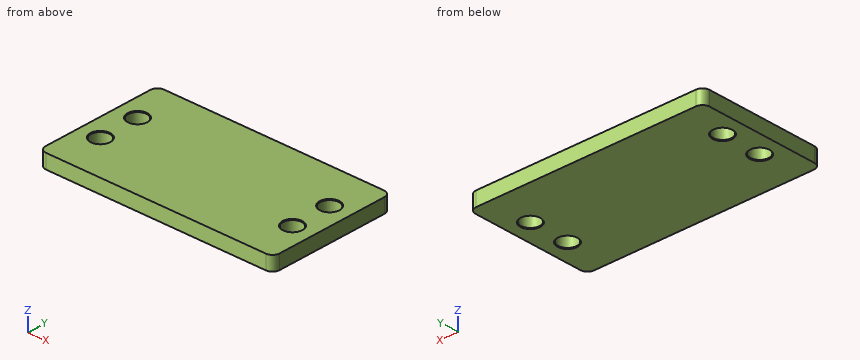
from build123d import *

# Parameters (mm, degrees)
SKETCH1_W                                 = 104.775
SKETCH1_H                                 = 57.15
BOSS_EXTRUDE1_DEPTH                       = 6.35
F_21_64_0_32813_DIAMETER_HOLE1_AT_2_COUNT = 2
F_21_64_0_32813_DIAMETER_HOLE1_AT_2_PITCH = 18
FILLET1_R                                 = 3.175


with BuildPart() as part:
    # Sketch1 → Boss-Extrude1 (new body)
    with BuildSketch(Plane.XY):
        Rectangle(SKETCH1_W, SKETCH1_H)
    extrude(amount=-BOSS_EXTRUDE1_DEPTH)

    # Sketch2 → 21/64 (0.32813) Diameter Hole1 (revolve, cut)
    with BuildSketch(Plane(origin=(43.000000106, 9, 0), x_dir=(0, -1, 0), z_dir=(1, 0, 0))):
        Polygon((0, 0), (0, 6.35), (4.445, 6.35), (4.167251, 6.072251), (4.167251, 0.277749), (4.445, 0), align=None)
    f_21_64_0_32813_diameter_hole1 = revolve(axis=Axis((43.000000106, 9, 6.35), (0, 0, -1)), mode=Mode.SUBTRACT)

    # 21/64 (0.32813) Diameter Hole1 at 2: 21/64 (0.32813) Diameter Hole1 ×2
    with Locations(*[(0, -i * F_21_64_0_32813_DIAMETER_HOLE1_AT_2_PITCH, 0) for i in range(1, F_21_64_0_32813_DIAMETER_HOLE1_AT_2_COUNT)]):
        add(f_21_64_0_32813_diameter_hole1, mode=Mode.SUBTRACT)

    # Mirror1: 21/64 (0.32813) Diameter Hole1 across plane
    add(f_21_64_0_32813_diameter_hole1.mirror(Plane(origin=(0, 0, 0), x_dir=(0, 0, 1), z_dir=(1, 0, 0))), mode=Mode.SUBTRACT)

    # Mirror1 copy 1 sketch → Mirror1 copy 1 (revolve, cut)
    with BuildSketch(Plane(origin=(-43.000000106, -9, 0), x_dir=(0, -1, 0), z_dir=(-1, 0, 0))):
        Polygon((0, 0), (0, -6.35), (4.445, -6.35), (4.167251, -6.072251), (4.167251, -0.277749), (4.445, 0), align=None)
    revolve(axis=Axis((-43.000000106, -9, 6.35), (0, 0, 1)), mode=Mode.SUBTRACT)

    # Fillet1
    fillet1_edges = [part.edges().sort_by_distance(p)[0] for p in [
        (-52.3875, 28.575, -3.175),
        (52.3875, 28.575, -3.175),
        (52.3875, -28.575, -3.175),
        (-52.3875, -28.575, -3.175),
    ]]
    fillet(fillet1_edges, radius=FILLET1_R)


solid = part.part
Part model, mm, in its own coordinate system. Coordinates: 2 decimals unless noted, no trailing zeros. Order: outer loops, then holes, each group sorted by start corner. A loop starts at its lowest first (then second) coordinate and runs counter-clockwise, first axis right, second up. Notation, with made-up numbers: M 55.25,64 L 62.25,64 A18 cw 62.25,85 Z; hole C 47.25,55 d4. An arc over 180 degrees is marked long. Use a Markdown table: item, result.
(1) Cut at B-B on x = 43. Write the cut outline in (y, z) (3 decimals), then the cut area to 3 significant figures.
A:
| item | result |
|---|---|
| outline | M -28.575,-6.35 L -13.445,-6.35 L -13.167,-6.072 L -13.167,-0.278 L -13.445,0 L -28.575,0 Z; M -4.833,-6.072 L -4.555,-6.35 L 4.555,-6.35 L 4.833,-6.072 L 4.833,-0.278 L 4.555,0 L -4.555,0 L -4.833,-0.278 Z; M 13.167,-6.072 L 13.445,-6.35 L 28.575,-6.35 L 28.575,0 L 13.445,0 L 13.167,-0.278 Z |
| area | 257 mm^2 |
(2) Cut at A-A on y = 9. State how many separate pieces and enclosed holes the cut face has, then the cut area to 3 significant figures.
A:
| item | result |
|---|---|
| separate pieces | 3 |
| enclosed holes | 0 |
| area | 559 mm^2 |
(3) Probe L1, parallel to X at y = 9, z = -2.5; L2, parallel to Y at x = -43, z = -2.9 (3 decimals); L3, parallel to X at y = 10.5, z = -3.25. List the from-to ranges inside material, lowest first.
A:
| item | result |
|---|---|
| L1 | x = -52.39 to -47.17, -38.83 to 38.83, 47.17 to 52.39 |
| L2 | y = -28.575 to -13.167, -4.833 to 4.833, 13.167 to 28.575 |
| L3 | x = -52.39 to -46.89, -39.11 to 39.11, 46.89 to 52.39 |
